The listing builds one solid part. Answer for the finished solid, in the listing's coordinates (mm). A direction names the side the tool comes from. Coordinates: 2 decimals unless noted, no trailing zeros. Write each loop counter-clockwise with the first axis right and the second up, starting at its lowest first coordinate (ties: lowest second). Pieces come first, ordered by that corner, then holes.
```python
from build123d import *

# Parameters (mm, degrees)
F0_R     = 2.199524
F1_DEPTH = 25.4


with BuildPart() as f1:
    # F0 (on Front) → F1 (new body)
    with BuildSketch(Plane.XZ):
        with BuildLine():
            ThreePointArc((-11.566241, 7.977341), (-9.949435, 9.043299), (-9.028414, 10.746839))
            ThreePointArc((-9.028414, 10.746839), (-8.936246, 11.233619), (-8.905364, 11.728085))
            ThreePointArc((-8.905364, 11.728085), (-16.120469, 14.027451), (-11.566241, 7.977341))
        make_face()
        with Locations((-12.879306, 11.728085)):
            Circle(F0_R, mode=Mode.SUBTRACT)
        with BuildLine():
            ThreePointArc((9.160321, 10.327597), (-0.017937, 6.897642), (-9.028414, 10.746839))
            ThreePointArc((-9.028414, 10.746839), (-9.949435, 9.043299), (-11.566241, 7.977341))
            ThreePointArc((-11.566241, 7.977341), (-7.823792, -0.003878), (-10.998232, -8.227545))
            ThreePointArc((-10.998232, -8.227545), (-9.468478, -9.688852), (-8.905364, -11.728085))
            ThreePointArc((-8.905364, -11.728085), (-8.909947, -11.918878), (-8.923684, -12.109232))
            ThreePointArc((-8.923684, -12.109232), (0.017868, -8.401069), (8.930846, -12.177395))
            ThreePointArc((8.930846, -12.177395), (9.331227, -9.938293), (10.894039, -8.285566))
            ThreePointArc((10.894039, -8.285566), (8.047392, -0.009584), (11.764413, 7.913739))
            ThreePointArc((11.764413, 7.913739), (10.177775, 8.813647), (9.160321, 10.327597))
        make_face()
        with BuildLine():
            ThreePointArc((16.853249, 11.728085), (12.167553, 15.637768), (9.160321, 10.327597))
            ThreePointArc((9.160321, 10.327597), (10.177775, 8.813647), (11.764413, 7.913739))
            ThreePointArc((11.764413, 7.913739), (15.26276, 8.548246), (16.853249, 11.728085))
        make_face()
        with Locations((12.879306, 11.728085)):
            Circle(F0_R, mode=Mode.SUBTRACT)
        with BuildLine():
            ThreePointArc((-8.905364, -11.728085), (-9.468478, -9.688852), (-10.998232, -8.227545))
            ThreePointArc((-10.998232, -8.227545), (-16.384108, -13.601207), (-8.923684, -12.109232))
            ThreePointArc((-8.923684, -12.109232), (-8.909947, -11.918878), (-8.905364, -11.728085))
        make_face()
        with Locations((-12.879306, -11.728085)):
            Circle(F0_R, mode=Mode.SUBTRACT)
        with BuildLine():
            ThreePointArc((16.853249, -11.728085), (14.867129, -8.287041), (10.894039, -8.285566))
            ThreePointArc((10.894039, -8.285566), (9.331227, -9.938293), (8.930846, -12.177395))
            ThreePointArc((8.930846, -12.177395), (13.104323, -15.695652), (16.853249, -11.728085))
        make_face()
        with Locations((12.879306, -11.728085)):
            Circle(F0_R, mode=Mode.SUBTRACT)
    extrude(amount=F1_DEPTH)


solid = f1.part
```
(1) Section D-D, the plane x = 3.5 is taken. Write down the section's boundary in (y, z), plus the area to 4 significant figures.
(2) Which of the six approach directions +Z, -Z, +X, -X, +Y, -Y give full straight-line access (tool end or side, diameter ignored) to faces 1 (the flat face through (0, 0, 0)), 2 (the cylindrical face through (-8.937, -12.522, 11.227))?
(3) Section B-B, the plane y = -8 is taken. Write down the section's boundary in (x, z), plus the area to 3 significant figures.
(4) Section C-C, the plane x = -14 is taken. Write down the section's boundary in (y, z), plus the area to 3 significant figures.
(5) Section A-A, the plane z = 12.5 is taken. Write down the section's boundary in (x, y).
(6) For a pull along X with two mould halves and no side action, classify faces 3 (the cylindrical face through (10.68, -12.52, 11.82)), 4 (the flat face through (0, -25.4, 0)) as pulls with the +X half, pulls with the -X half, needs draft (parallel to the pull), parting line crosses it, or undercut.
(7) Each of these flat-tipped pins is pushed along its axis until it touches: pin 1 (6 mm diameter, centred on x = -3, y = -10, fed in from +Z); pin 2 (2 mm diameter, centred on x = 8, z = 12, fed in from -Y); pin 3 (10 mm diameter, centred on y = -3, z = -2.5, fed in from -X); pin 4 (12 mm diameter, centred on y = -9, z = 2.5, fed in from +X). Where does it stop, or does it pass through?
(8) Find the intervals of material crossed by probe 1 along X at (y, z) = (-19, -11); probe 2 along Z at (x, y) = (13.5, -7.25); probe 3 along Z at (x, y) = (11.5, -12.5), in increasing order.
Solution:
1. outline: (-25.4, -8.91) - (0, -8.91) - (0, 7.29) - (-25.4, 7.29) - close
1. area: 411.5 mm2
2. face 1: +Z, -Z, +X, -X, +Y
2. face 2: +Y, -Y
3. outline: (-11.57, 7.98) arc R11.23 cw to (-11, -8.23) arc R3.97 ccw (long way) to (-8.92, -12.11) arc R12.52 cw to (8.93, -12.18) arc R3.97 ccw (long way) to (10.89, -8.29) arc R11.65 cw to (11.76, 7.91) arc R3.97 ccw to (16.85, 11.73) arc R3.97 ccw (long way) to (9.16, 10.33) arc R13.19 cw to (-9.03, 10.75) arc R3.97 ccw to (-8.91, 11.73) arc R3.97 ccw (long way) to start; hole circle Ø4.4 at (-12.88, -11.73); hole circle Ø4.4 at (-12.88, 11.73); hole circle Ø4.4 at (12.88, -11.73); hole circle Ø4.4 at (12.88, 11.73)
3. area: 462 mm2
4. outline: (-25.4, -15.54) - (0, -15.54) - (0, -13.62) - (-25.4, -13.62) - close; (-25.4, -9.84) - (0, -9.84) - (0, -7.92) - (-25.4, -7.92) - close; (-25.4, 7.92) - (0, 7.92) - (0, 9.84) - (-25.4, 9.84) - close; (-25.4, 13.62) - (0, 13.62) - (0, 15.54) - (-25.4, 15.54) - close
4. area: 195 mm2
5. outline: (-16.78, -25.4) - (-14.94, -25.4) - (-14.94, 0) - (-16.78, 0) - close; (-10.82, -25.4) - (-8.98, -25.4) - (-8.98, 0) - (-10.82, 0) - close; (8.98, -25.4) - (10.82, -25.4) - (10.82, 0) - (8.98, 0) - close; (14.94, -25.4) - (16.78, -25.4) - (16.78, 0) - (14.94, 0) - close
6. face 3: undercut
6. face 4: needs draft
7. pin 1: stops at z = 8.49
7. pin 2: stops at y = -25.4
7. pin 3: stops at x = -10.35
7. pin 4: stops at x = 15.2
8. probe 1: x = -16.79 to -14.95, -10.8 to -7.67, 7.61 to 10.8, 14.95 to 16.79
8. probe 2: z = -15.65 to -13.84, -9.62 to -7.8, 7.8 to 9.62, 13.84 to 15.65
8. probe 3: z = -15.45 to -13.44, -10.01 to -8, 7.66 to 10.01, 13.44 to 15.45
